Build history of the part. All positions in model axes, mm. A direction names the side the tool comes from. Coordinates: 2 decimals unless noted, no trailing zeros. Order: outer loops, then holes, each group sorted by start corner. A loop starts at its lowest first (then second) coordinate and runs counter-clockwise, first axis right, second up. Notation, with made-up numbers: M -34,26.25 L -22,26.25 A26 cw -22,47.25 Z; hole C -20,-13 d10. An arc over 180 degrees is marked long. Use a Markdown table: item, result. Add a question column.
from build123d import *

# Parameters (mm, degrees)
SKETCH1_W           = 122
SKETCH1_H           = 112
BOSS_EXTRUDE1_DEPTH = 6.2
SKETCH2_W           = 100
SKETCH2_H           = 70
BOSS_EXTRUDE2_DEPTH = 6.2
SKETCH3_R           = 1.25
SKETCH3_R_2         = 1.65
SKETCH3_R_3         = 15
CUT_EXTRUDE1_DEPTH  = 141.126514265
SKETCH4_R           = 1.55
SKETCH4_R_2         = 1.65
CUT_EXTRUDE2_DEPTH  = 141.126514265
SKETCH5_R           = 2
CUT_EXTRUDE3_DEPTH  = 10
SKETCH6_R           = 5
CUT_EXTRUDE4_DEPTH  = 10
SKETCH7_R           = 2.25
CUT_EXTRUDE5_DEPTH  = 141.126514265


with BuildPart() as part:
    # Sketch1 → Boss-Extrude1 (new body)
    with BuildSketch(Plane(origin=(0, 0, 0), x_dir=(1, 0, 0), z_dir=(0, 1, 0))):
        Rectangle(SKETCH1_W, SKETCH1_H)
    extrude(amount=BOSS_EXTRUDE1_DEPTH)

    # Sketch2 → Boss-Extrude2 (add)
    with BuildSketch(Plane(origin=(0, 0, 0), x_dir=(1, 0, 0), z_dir=(0, 1, 0))):
        with Locations((0, 91)):
            Rectangle(SKETCH2_W, SKETCH2_H)
    extrude(amount=BOSS_EXTRUDE2_DEPTH)

    # Sketch3 → Cut-Extrude1 (cut, through all)
    with BuildSketch(Plane(origin=(0, 6.2, 0), x_dir=(1, 0, 0), z_dir=(0, 1, 0))):
        with Locations(Location((-46.5, 61, 0), (0, 0, 270))):
            Circle(SKETCH3_R)
        with Locations(Location((-24.5, 61, 0), (0, 0, 270))):
            Circle(SKETCH3_R)
        with Locations(Location((-46.013, 106, 0), (0, 0, 270))):
            Circle(SKETCH3_R_2)
        with Locations(Location((0, 99, 0), (0, 0, 270))):
            Circle(SKETCH3_R_3)
        with Locations(Location((-46.013, 92, 0), (0, 0, 270))):
            Circle(SKETCH3_R_2)
        with Locations(Location((46.013, 92, 0), (0, 0, 270))):
            Circle(SKETCH3_R_2)
        with Locations(Location((46.013, 106, 0), (0, 0, 270))):
            Circle(SKETCH3_R_2)
    extrude(amount=-CUT_EXTRUDE1_DEPTH, mode=Mode.SUBTRACT)

    # Sketch4 → Cut-Extrude2 (cut, through all)
    with BuildSketch(Plane(origin=(0, 6.2, 0), x_dir=(1, 0, 0), z_dir=(0, 1, 0))):
        with Locations(Location((-49.5, 51, 0), (0, 0, 270))):
            Circle(SKETCH4_R)
        with Locations(Location((-49.5, 43, 0), (0, 0, 270))):
            Circle(SKETCH4_R)
        with Locations(Location((-14, 2.5, 0), (0, 0, 270))):
            Circle(SKETCH4_R_2)
        with Locations(Location((14, 2.5, 0), (0, 0, 270))):
            Circle(SKETCH4_R_2)
        with Locations(Location((14, -5.5, 0), (0, 0, 270))):
            Circle(SKETCH4_R_2)
        with Locations(Location((-14, -5.5, 0), (0, 0, 270))):
            Circle(SKETCH4_R_2)
        with Locations(Location((-14, 51, 0), (0, 0, 270))):
            Circle(SKETCH4_R_2)
        with Locations(Location((14, 51, 0), (0, 0, 270))):
            Circle(SKETCH4_R_2)
        with Locations(Location((14, 43, 0), (0, 0, 270))):
            Circle(SKETCH4_R_2)
        with Locations(Location((-14, 43, 0), (0, 0, 270))):
            Circle(SKETCH4_R_2)
        with Locations(Location((49.5, 43, 0), (0, 0, 270))):
            Circle(SKETCH4_R)
        with Locations(Location((49.5, 51, 0), (0, 0, 270))):
            Circle(SKETCH4_R)
    extrude(amount=-CUT_EXTRUDE2_DEPTH, mode=Mode.SUBTRACT)

    # Sketch5 → Cut-Extrude3 (cut)
    with BuildSketch(Plane(origin=(0, 6.2, 0), x_dir=(1, 0, 0), z_dir=(0, 1, 0))):
        with Locations(Location((-53, 31, 0), (0, 0, 270))):
            Circle(SKETCH5_R)
        with Locations(Location((-53, 16, 0), (0, 0, 270))):
            Circle(SKETCH5_R)
        with Locations(Location((53, 16, 0), (0, 0, 270))):
            Circle(SKETCH5_R)
        with Locations(Location((53, 31, 0), (0, 0, 270))):
            Circle(SKETCH5_R)
    extrude(amount=-CUT_EXTRUDE3_DEPTH, mode=Mode.SUBTRACT)

    # Sketch6 → Cut-Extrude4 (cut)
    with BuildSketch(Plane(origin=(0, 6.2, 0), x_dir=(1, 0, 0), z_dir=(0, 1, 0))):
        with Locations(Location((-28.75, -27.5, 0), (0, 0, 270))):
            Circle(SKETCH6_R)
        with Locations(Location((28.75, -27.5, 0), (0, 0, 270))):
            Circle(SKETCH6_R)
    extrude(amount=-CUT_EXTRUDE4_DEPTH, mode=Mode.SUBTRACT)

    # Sketch7 → Cut-Extrude5 (cut, through all)
    with BuildSketch(Plane(origin=(0, 6.2, 0), x_dir=(1, 0, 0), z_dir=(0, 1, 0))):
        with Locations(Location((-56, -36, 0), (0, 0, 270))):
            Circle(SKETCH7_R)
        with Locations(Location((-56, -46, 0), (0, 0, 270))):
            Circle(SKETCH7_R)
        with Locations(Location((56, -46, 0), (0, 0, 270))):
            Circle(SKETCH7_R)
        with Locations(Location((56, -36, 0), (0, 0, 270))):
            Circle(SKETCH7_R)
    extrude(amount=-CUT_EXTRUDE5_DEPTH, mode=Mode.SUBTRACT)


solid = part.part
(1) Slice it at C-C on z = -31. Give the cut face in (x, y), and give its area (3 significant figures).
(2) Drop flat-ended pins along their axis: P1, Ø6, axis at x = 28.75, z = 27.5, coming from the -Y side; P2, Ø3, axis at x = 57.5, y = 4, coming from the -Z side. Give the stop position or say it passes through.
(3) Drill centre lines: line 1 along X through (y, z) = (4.75, -43); line 2 along X through (y, z) = (4.5, 36); line 3 along X through (y, z) = (3, 5.5). Where is each one in solid material? Low to high. Write a range as from..to.
(4) Slice it at D-D on y = 3. State how many separate pieces and enclosed holes the cut face has, and give its area (3 significant figures).
(5) Which spindle directions (+Z, -Z, +X, -X, +Y, -Y) get a long thin tool onto all of the face, cutting with end or side? Do faces 1 (the flat face through (50, 3, -91)), 2 (the cylindrical face through (-47.017, 3.143, -107.309)). Say none if no direction does.
(6) Slice it at B-B on z = -95.5. Give the cut face in (x, y), and give its area (3 significant figures).
(7) Slice it at A-A on z = 27.5. Give the cut face in (x, y), and give its area (3 significant figures).
(8) Mould opens along Z. For faces 3 (the flat face through (55, 3, -56)), 4 (the cylindrical face through (-12.61, 3.14, -50.11)), 5 (the flat face through (-1, 0, -36)) say: released by +Z, released by -Z, zero draft, split by the parting line, or undercut.
Solutions:
| question | item | result |
|---|---|---|
| 1 | outline | M -61,0 L -55,0 L -55,6.2 L -61,6.2 Z; M -51,0 L 51,0 L 51,6.2 L -51,6.2 Z; M 55,0 L 61,0 L 61,6.2 L 55,6.2 Z |
| 1 | area | 707 mm² |
| 2 | P1 | through |
| 2 | P2 | z = -56 |
| 3 | line 1 | -61..-51.05, -47.95..-15.65, -12.35..12.35, 15.65..47.95, 51.05..61 |
| 3 | line 2 | -61..-58.25, -53.75..53.75, 58.25..61 |
| 3 | line 3 | -61..-15.65, -12.35..12.35, 15.65..61 |
| 4 | separate pieces | 1 |
| 4 | enclosed holes | 29 |
| 4 | area | 19,500 mm² |
| 5 | face 1 | -Z, +X, +Y, -Y |
| 5 | face 2 | +Y, -Y |
| 6 | outline | M -50,0 L -14.59,0 L -14.59,6.2 L -50,6.2 Z; M 14.59,0 L 50,0 L 50,6.2 L 14.59,6.2 Z |
| 6 | area | 439 mm² |
| 7 | outline | M -61,0 L -33.75,0 L -33.75,6.2 L -61,6.2 Z; M -23.75,0 L 23.75,0 L 23.75,6.2 L -23.75,6.2 Z; M 33.75,0 L 61,0 L 61,6.2 L 33.75,6.2 Z |
| 7 | area | 632 mm² |
| 8 | face 3 | released by -Z |
| 8 | face 4 | undercut |
| 8 | face 5 | zero draft |
